```python
from build123d import *

# Parameters (mm, degrees)
F0_W     = 25
F0_H     = 20
F1_DEPTH = 25
F2_W     = 10
F2_H     = 10
F3_DEPTH = 10
F4_R     = 2.5
F5_DEPTH = 10


with BuildPart() as f1:
    # F0 (on Top) → F1 (new body)
    with BuildSketch(Plane.XY):
        Rectangle(F0_W, F0_H)
    extrude(amount=F1_DEPTH)

    # F2 (on face) → F3 (join)
    with BuildSketch(Plane(origin=(0, 10, 0), x_dir=(-1, 0, 0), z_dir=(0, 1, 0))):
        with Locations((0, 12.5)):
            Rectangle(F2_W, F2_H)
    extrude(amount=F3_DEPTH)

    # F4 (on face) → F5 (cut, through all)
    with BuildSketch(Plane(origin=(0, 20, 0), x_dir=(-1, 0, 0), z_dir=(0, 1, 0))):
        with Locations((0, 12.5)):
            Circle(F4_R)
    extrude(amount=-F5_DEPTH, mode=Mode.SUBTRACT)


solid = f1.part
```
Can you work these out from the model? Positions are in its coordinate system, mm. A direction names the side the tool comes from. Give positions to 0.01 mm unless a question says otherwise; leave off trailing zeros. Loops run counter-clockwise (first coordinate to the right, second up) from the corner with the lowest first, then second, coordinate; pieces in that order, holes last. Notation, with made-up numbers: M 15.5,36 L 35.5,36 A13 cw 35.5,46 Z; hole C 41.25,81.25 d2. An arc over 180 degrees is marked long. Use CSV: the item, a comma, the result in double quotes. Start each with the question number.
1. Imagine slicing it at B-B, the plane z = 12.5. Write out the boundary of the cut face in (x, y).
2. For P1, Ø11, axis at y = 16.5, z = 11.5, coming from the -X side; P2, Ø5, axis at x = 1, y = 14.5, coming from the +Z side; P3, Ø4, axis at x = 0, z = 12.5, coming from the +Y side, each with a flat end and sliding along its axis, tell me the tip position at first contact or that it passes through.
3. Imagine slicing it at A-A, the plane x = 0. Write out the boundary of the cut face in (y, z).
4. If we mould it in two halves opening along Z, with no side actions, what happens to faces 5 (the face through (0, -10, 12)), 6 (the face through (0, 0, 0)), 7 (the face through (0.54, 15.07, 10.06))? For each: released by +Z, released by -Z, zero draft, split by the parting line, or undercut.
5. Imagine slicing it at D-D, the plane z = 8.5. Write out the boundary of the cut face in (x, y), plus the area to 3 significant figures.
6. On a 3-axis mill with a long thin cutter (end or side, diameter ignored), from which of +Z, -Z, +X, -X, +Y, -Y can I reach the whole of each face in a straight line? I mean faces 1 (the face through (-5, 15, 12)), 2 (the face through (0, 15, 17.5)), 3 (the face through (5, 15, 12)), 4 (the face through (0, 10, 13)). Say none if no direction works.
7. Imagine slicing it at C-C, the plane y = 16.25. Write out the boundary of the cut face in (x, z).
8. If I drill on L1, parallel to Z at x = 0, y = 17.75; L2, parallel to Y at x = -6.5, z = 19.5; L3, parallel to Z at x = -3.75, y = 15.25, over which ranges is the centre line in solid material (lowest first)?
Response values:
1,outline,"M -12.5,-10 L 12.5,-10 L 12.5,10 L 5,10 L 5,20 L 2.5,20 L 2.5,10 L -2.5,10 L -2.5,20 L -5,20 L -5,10 L -12.5,10 Z"
2,P1,"x = -5"
2,P2,"z = 17.5"
2,P3,"y = 10"
3,outline,"M -10,0 L 10,0 L 10,7.5 L 20,7.5 L 20,10 L 10,10 L 10,15 L 20,15 L 20,17.5 L 10,17.5 L 10,25 L -10,25 Z"
4,face 5,"zero draft"
4,face 6,"released by -Z"
4,face 7,"undercut"
5,outline,"M -12.5,-10 L 12.5,-10 L 12.5,10 L 5,10 L 5,20 L -5,20 L -5,10 L -12.5,10 Z"
5,area,"600 mm^2"
6,face 1,"+Z, -Z, -X, +Y"
6,face 2,"+Z, +X, -X, +Y"
6,face 3,"+Z, -Z, +X, +Y"
6,face 4,"+Y"
7,outline,"M -5,7.5 L 5,7.5 L 5,17.5 L -5,17.5 Z; hole C 0,12.5 d5"
8,L1,"7.5 to 10, 15 to 17.5"
8,L2,"-10 to 10"
8,L3,"7.5 to 17.5"
